Geometry: final body of the model. Coordinates: model frame, mm. Coordinates: 2 decimals unless noted, no trailing zeros. Loops run counter-clockwise (first coordinate to the right, second up) from the corner with the lowest first, then second, coordinate; pieces in that order, holes last. Notation, with made-up numbers: (86, 28) - (104, 28) arc R34 ccw to (104, 64) - close; hole circle Ø1 at (-15, 32.5). An arc over 180 degrees is marked (long way). Put each result on its own line as item: value. Start each with the question number.
1) Material intervals for line 1 along X through (y, z) = (24.5, 5); line 2 along Y through (x, z) = (-4, 9.25), sorted ascending. Write a range as from..to.
2) Section A-A on y = 14.5. Output: boundary loops of the cut face in (x, z), and give its area (3 significant figures).
3) Section C-C on x = 11. Output: boundary loops of the cut face in (y, z), and give its area (3 significant figures).
4) Section B-B on y = -19.5. Count the separate pieces of the cut face and the enclosed holes in it, and give its area (3 significant figures).
```python
from build123d import *

# Parameters (mm, degrees)
F0_W     = 7.6
F0_H     = 7.6
F1_DEPTH = 10


with BuildPart() as f1:
    # F0 (on Top) → F1 (new body)
    with BuildSketch(Plane.XY):
        Polygon((29.8, 29.8), (0, 29.8), (-29.8, 29.8), (-29.8, 0), (-29.8, -29.8), (0, -29.8), (29.8, -29.8), (29.8, 0), align=None)
        with Locations((-25.2, -25.2)):
            Rectangle(F0_W, F0_H, mode=Mode.SUBTRACT)
        with Locations((-16.8, -25.2)):
            Rectangle(F0_W, F0_H, mode=Mode.SUBTRACT)
        with Locations((-25.2, -16.8)):
            Rectangle(F0_W, F0_H, mode=Mode.SUBTRACT)
        with Locations((-16.8, -16.8)):
            Rectangle(F0_W, F0_H, mode=Mode.SUBTRACT)
        with Locations((-8.4, -25.2)):
            Rectangle(F0_W, F0_H, mode=Mode.SUBTRACT)
        with Locations((-8.4, -16.8)):
            Rectangle(F0_W, F0_H, mode=Mode.SUBTRACT)
        with Locations((-25.2, -8.4)):
            Rectangle(F0_W, F0_H, mode=Mode.SUBTRACT)
        with Locations((-16.8, -8.4)):
            Rectangle(F0_W, F0_H, mode=Mode.SUBTRACT)
        with Locations((-8.4, -8.4)):
            Rectangle(F0_W, F0_H, mode=Mode.SUBTRACT)
        Polygon((0, -29), (-3.8, -29), (-3.8, -21.4), (0, -21.4), (3.8, -21.4), (3.8, -29), align=None, mode=Mode.SUBTRACT)
        with Locations((8.4, -25.2)):
            Rectangle(F0_W, F0_H, mode=Mode.SUBTRACT)
        Polygon((0, -20.6), (-3.8, -20.6), (-3.8, -13), (0, -13), (3.8, -13), (3.8, -20.6), align=None, mode=Mode.SUBTRACT)
        with Locations((8.4, -16.8)):
            Rectangle(F0_W, F0_H, mode=Mode.SUBTRACT)
        with Locations((16.8, -25.2)):
            Rectangle(F0_W, F0_H, mode=Mode.SUBTRACT)
        with Locations((25.2, -25.2)):
            Rectangle(F0_W, F0_H, mode=Mode.SUBTRACT)
        with Locations((16.8, -16.8)):
            Rectangle(F0_W, F0_H, mode=Mode.SUBTRACT)
        with Locations((25.2, -16.8)):
            Rectangle(F0_W, F0_H, mode=Mode.SUBTRACT)
        Polygon((0, -12.2), (-3.8, -12.2), (-3.8, -4.6), (0, -4.6), (3.8, -4.6), (3.8, -12.2), align=None, mode=Mode.SUBTRACT)
        with Locations((8.4, -8.4)):
            Rectangle(F0_W, F0_H, mode=Mode.SUBTRACT)
        with Locations((16.8, -8.4)):
            Rectangle(F0_W, F0_H, mode=Mode.SUBTRACT)
        with Locations((25.2, -8.4)):
            Rectangle(F0_W, F0_H, mode=Mode.SUBTRACT)
        with Locations((-25.2, 0)):
            Rectangle(F0_W, F0_H, mode=Mode.SUBTRACT)
        with Locations((-16.8, 0)):
            Rectangle(F0_W, F0_H, mode=Mode.SUBTRACT)
        with Locations((-25.2, 8.4)):
            Rectangle(F0_W, F0_H, mode=Mode.SUBTRACT)
        with Locations((-16.8, 8.4)):
            Rectangle(F0_W, F0_H, mode=Mode.SUBTRACT)
        with Locations((-8.4, 0)):
            Rectangle(F0_W, F0_H, mode=Mode.SUBTRACT)
        with Locations((-8.4, 8.4)):
            Rectangle(F0_W, F0_H, mode=Mode.SUBTRACT)
        Polygon((0, -3.8), (-3.8, -3.8), (-3.8, 3.8), (0, 3.8), (3.8, 3.8), (3.8, -3.8), align=None, mode=Mode.SUBTRACT)
        with Locations((8.4, 0)):
            Rectangle(F0_W, F0_H, mode=Mode.SUBTRACT)
        Polygon((-3.8, 4.6), (-3.8, 12.2), (0, 12.2), (3.8, 12.2), (3.8, 4.6), (0, 4.6), align=None, mode=Mode.SUBTRACT)
        with Locations((8.4, 8.4)):
            Rectangle(F0_W, F0_H, mode=Mode.SUBTRACT)
        with Locations((16.8, 0)):
            Rectangle(F0_W, F0_H, mode=Mode.SUBTRACT)
        with Locations((25.2, 0)):
            Rectangle(F0_W, F0_H, mode=Mode.SUBTRACT)
        with Locations((16.8, 8.4)):
            Rectangle(F0_W, F0_H, mode=Mode.SUBTRACT)
        with Locations((25.2, 8.4)):
            Rectangle(F0_W, F0_H, mode=Mode.SUBTRACT)
        Polygon((0, 13), (-29, 13), (-29, 29), (0, 29), (29, 29), (29, 13), align=None, mode=Mode.SUBTRACT)
    extrude(amount=F1_DEPTH)


solid = f1.part
```
Answer block:
1. line 1: x = -29.8..-29, 29..29.8
1. line 2: y = -29.8..13, 29..29.8
2. outline: (-29.8, 0) - (-29, 0) - (-29, 10) - (-29.8, 10) - close; (29, 0) - (29.8, 0) - (29.8, 10) - (29, 10) - close
2. area: 16.0 mm²
3. outline: (-29.8, 0) - (-29, 0) - (-29, 10) - (-29.8, 10) - close; (-21.4, 0) - (-20.6, 0) - (-20.6, 10) - (-21.4, 10) - close; (-13, 0) - (-12.2, 0) - (-12.2, 10) - (-13, 10) - close; (-4.6, 0) - (-3.8, 0) - (-3.8, 10) - (-4.6, 10) - close; (3.8, 0) - (4.6, 0) - (4.6, 10) - (3.8, 10) - close; (12.2, 0) - (13, 0) - (13, 10) - (12.2, 10) - close; (29, 0) - (29.8, 0) - (29.8, 10) - (29, 10) - close
3. area: 56.0 mm²
4. separate pieces: 8
4. enclosed holes: 0
4. area: 64.0 mm²
